Part print with two shaded views. Sizes in mm from the minimum x, y, z corner. Round coordinates to 2 decimals unless told otherwise and drop trailing zeros. Write each loop counter-clockwise with the first axis right and the second up, starting at its lowest first coordinate (ties: lowest second). Pieces come first, ordered by that corner, then holes. Notation, with made-up numbers: (-14.75, 63) -> (-5.75, 63) arc R18 cw to (-5.75, 82) -> close; hole circle Ø10 at (8.25, 10). An arc over 180 degrees is marked (long way). Answer in a Markdown table with one row per item.
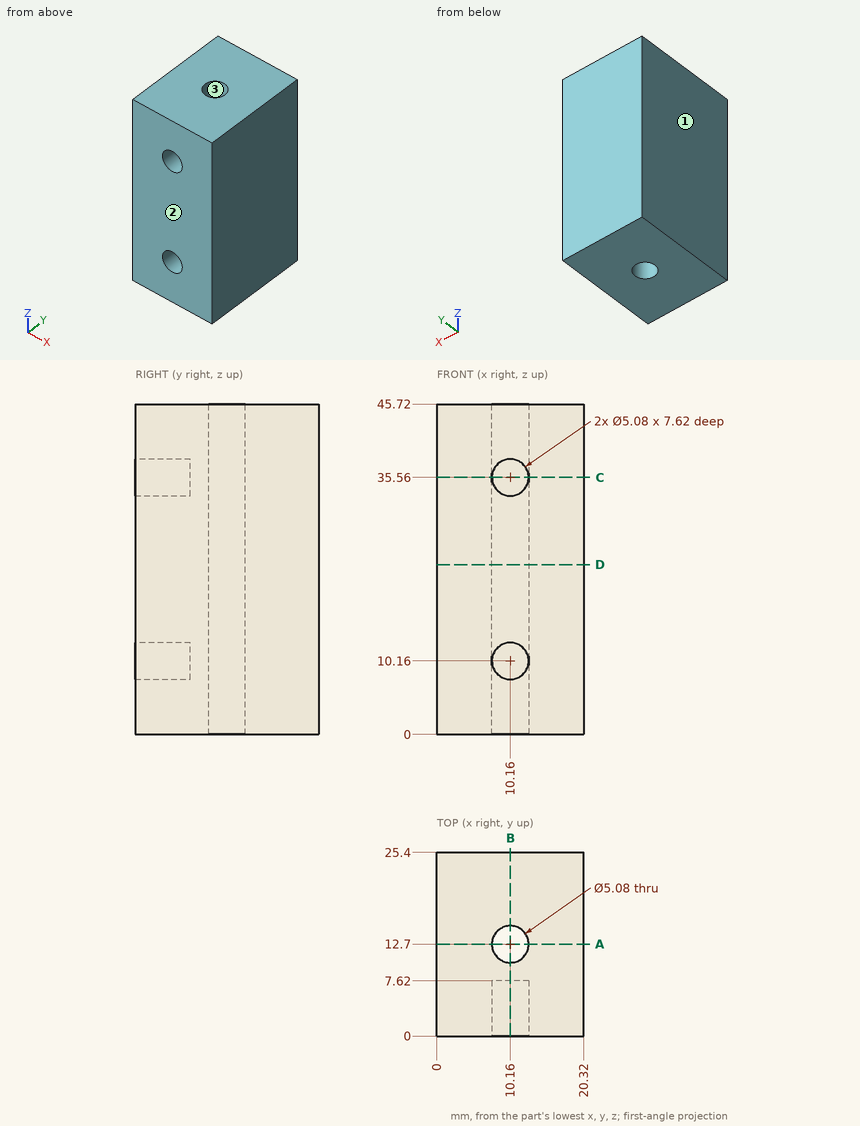
Q1. Wall check: line 1 (Y direction, x = 10, z = 5.5); line 2 (Z direction, x = 8, y = 2.75); line 3 (Y direction, x = 10.16, z = 12). Give the ranges that are in metal, low to high. Write a range as [from, to].
A:
| item | result |
|---|---|
| line 1 | [0, 10.17], [15.23, 25.4] |
| line 2 | [0, 8.82], [11.5, 34.22], [36.9, 45.72] |
| line 3 | [7.62, 10.16], [15.24, 25.4] |
Q2. Drop a flat-ended pin along its axis: P1, Ø2.5, axis at x = 10, z = 10, coming from the -Y side. Give the stop position or say it passes through.
A:
| item | result |
|---|---|
| P1 | y = 7.62 |
Q3. Saw through at D-D on z = 23.5. Write the cut outline in (x, y).
A:
| item | result |
|---|---|
| outline | (0, 0) -> (20.32, 0) -> (20.32, 25.4) -> (0, 25.4) -> close; hole circle Ø5.08 at (10.16, 12.7) |
Q4. Saw through at C-C on z = 35.56. Write the cut outline in (x, y), plus the area to 3 significant figures.
A:
| item | result |
|---|---|
| outline | (0, 0) -> (7.62, 0) -> (7.62, 7.62) -> (12.7, 7.62) -> (12.7, 0) -> (20.32, 0) -> (20.32, 25.4) -> (0, 25.4) -> close; hole circle Ø5.08 at (10.16, 12.7) |
| area | 457 mm² |
Q5. Saw through at B-B on x = 10.16. Write the cut outline in (y, z).
A:
| item | result |
|---|---|
| outline | (0, 0) -> (10.16, 0) -> (10.16, 45.72) -> (0, 45.72) -> (0, 38.1) -> (7.62, 38.1) -> (7.62, 33.02) -> (0, 33.02) -> (0, 12.7) -> (7.62, 12.7) -> (7.62, 7.62) -> (0, 7.62) -> close; (15.24, 0) -> (25.4, 0) -> (25.4, 45.72) -> (15.24, 45.72) -> close |
Q6. Two-plate mould, pull along X, no slides. Class the marked faces 1, 2 and 3: released by +X, released by -X, zero draft, split by the parting line, or undercut.
A:
| item | result |
|---|---|
| face 1 | released by -X |
| face 2 | zero draft |
| face 3 | undercut |
Q7. Saw through at A-A on y = 12.7. Write the cut outline in (x, z).
A:
| item | result |
|---|---|
| outline | (0, 0) -> (7.62, 0) -> (7.62, 45.72) -> (0, 45.72) -> close; (12.7, 0) -> (20.32, 0) -> (20.32, 45.72) -> (12.7, 45.72) -> close |
